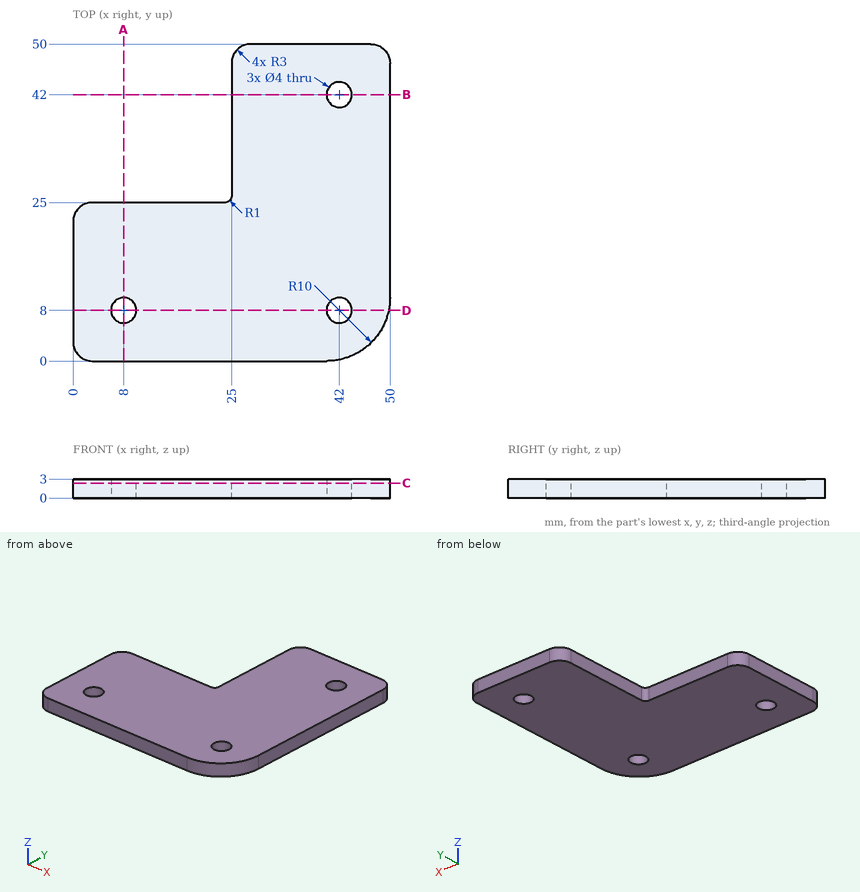
Input: dimensioned drawing with shaded views. Units: mm. Origin: part minimum x, y, z. Give positions to 0.01 mm unless a question says otherwise; leave off trailing zeros. Loops run counter-clockwise (first coordinate to the right, second up) from the corner with the lowest first, then second, coordinate; pieces in that order, holes last. Notation, with made-up numbers: (-27, 78) -> (-14, 78) arc R30 ccw to (-14, 112) -> close; hole circle Ø5 at (13.25, 5). An arc over 180 degrees is marked (long way). Use a Markdown table: item, result.
Q1. Section query D-D, the plane y = 8. Return the cut outline in (x, z), plus the area to 3 significant figures.
Entries:
| item | result |
|---|---|
| outline | (0, 0) -> (6, 0) -> (6, 3) -> (0, 3) -> close; (10, 0) -> (40, 0) -> (40, 3) -> (10, 3) -> close; (44, 0) -> (49.8, 0) -> (49.8, 3) -> (44, 3) -> close |
| area | 125 mm² |
Q2. Section query B-B, the plane y = 42. Return the cut outline in (x, z).
Entries:
| item | result |
|---|---|
| outline | (25, 0) -> (40, 0) -> (40, 3) -> (25, 3) -> close; (44, 0) -> (50, 0) -> (50, 3) -> (44, 3) -> close |
Q3. First-contact query: P1, Ø3.5, axis at x = 42, y = 42, coming from the -Z side. Flat tip, straight axial feed; report the tip coordinate or a pass-through.
Entries:
| item | result |
|---|---|
| P1 | passes through |
Q4. Section query A-A, the plane x = 8. Return the cut outline in (y, z), plus the area to 3 significant figures.
Entries:
| item | result |
|---|---|
| outline | (0, 0) -> (6, 0) -> (6, 3) -> (0, 3) -> close; (10, 0) -> (25, 0) -> (25, 3) -> (10, 3) -> close |
| area | 63.0 mm² |
Q5. Section query C-C, the plane z = 2.35. Return the cut outline in (x, y), plus the area to 3 significant figures.
Entries:
| item | result |
|---|---|
| outline | (0, 3) arc R3 ccw to (3, 0) -> (40, 0) arc R10 ccw to (50, 10) -> (50, 47) arc R3 ccw to (47, 50) -> (28, 50) arc R3 ccw to (25, 47) -> (25, 26) arc R1 cw to (24, 25) -> (3, 25) arc R3 ccw to (0, 22) -> close; hole circle Ø4 at (8, 8); hole circle Ø4 at (42, 8); hole circle Ø4 at (42, 42) |
| area | 1,810 mm² |
Q6. Ray query, probe 1 along Y at (x, z) = (42, 1.9); probe 2 along X at (y, z) = (42, 0.9); probe 3 along X at (y, z) = (8, 1.4). Return the intervals inside material, ascending. Write a range as from..to.
Entries:
| item | result |
|---|---|
| probe 1 | y = 0.2..6, 10..40, 44..50 |
| probe 2 | x = 25..40, 44..50 |
| probe 3 | x = 0..6, 10..40, 44..49.8 |
